Design review of the part built by this model. Coordinates are the model's own, in mm. A direction names the side the tool comes from. Round coordinates to 2 decimals unless told otherwise and drop trailing zeros. Loops run counter-clockwise (first coordinate to the right, second up) from the corner with the lowest first, then second, coordinate; pieces in that order, holes last. Notation, with made-up numbers: M 60.5,3.5 L 102.5,3.5 A21 cw 102.5,40.5 Z; hole C 84,-23.5 d9. An arc over 180 degrees is marked long. Use a Markdown table: item, result.
from build123d import *

# Parameters (mm, degrees)
SKETCH1_R           = 16
BOSS_EXTRUDE1_DEPTH = 12.5
SKETCH2_R           = 15
CUT_EXTRUDE1_DEPTH  = 10
SKETCH3_R           = 5
CUT_EXTRUDE2_DEPTH  = 10
SKETCH4_R           = 1
CUT_EXTRUDE3_DEPTH  = 10


with BuildPart() as part:
    # Sketch1 → Boss-Extrude1 (new body)
    with BuildSketch(Plane(origin=(0, 0, 0), x_dir=(1, 0, 0), z_dir=(0, 1, 0))):
        with Locations(Location((0, 0, 0), (0, 0, 270))):
            Circle(SKETCH1_R)
    extrude(amount=BOSS_EXTRUDE1_DEPTH)

    # Sketch2 → Cut-Extrude1 (cut)
    with BuildSketch(Plane(origin=(0, 12.5, 0), x_dir=(1, 0, 0), z_dir=(0, 1, 0))):
        with Locations(Location((0, 0, 0), (0, 0, 270))):
            Circle(SKETCH2_R)
    extrude(amount=-CUT_EXTRUDE1_DEPTH, mode=Mode.SUBTRACT)

    # Sketch3 → Cut-Extrude2 (cut)
    with BuildSketch(Plane(origin=(0, 0, 0), x_dir=(-1, 0, 0), z_dir=(0, -1, 0))):
        with Locations(Location((0, 0, 0), (0, 0, 90))):
            Circle(SKETCH3_R)
    extrude(amount=-CUT_EXTRUDE2_DEPTH, mode=Mode.SUBTRACT)

    # Sketch4 → Cut-Extrude3 (cut)
    with BuildSketch(Plane(origin=(0, 0, 0), x_dir=(-1, 0, 0), z_dir=(0, -1, 0))):
        with Locations(Location((0, 8, 0), (0, 0, 90))):
            Circle(SKETCH4_R)
        with Locations(Location((0, -8, 0), (0, 0, 90))):
            Circle(SKETCH4_R)
        with Locations(Location((-8, 0, 0), (0, 0, 90))):
            Circle(SKETCH4_R)
        with Locations(Location((8, 0, 0), (0, 0, 90))):
            Circle(SKETCH4_R)
    extrude(amount=-CUT_EXTRUDE3_DEPTH, mode=Mode.SUBTRACT)


solid = part.part
1. Insertion check: pin 1 (4 mm diameter, centred on x = 2.5, z = 7.5, fed in from +Y); pin 2 (6 mm diameter, centred on y = 4, z = 11, fed in from +X); pin 3 (1.2 mm diameter, centred on x = 0, z = 8, fed in from +Y); pin 4 (1.5 mm diameter, centred on x = -7.5, y = 9, fed in from +Z). Each pin has a flat end and moves straight along its axis. Give the tip position at first contact, or say it passes through.
Check values:
| item | result |
|---|---|
| pin 1 | stops at y = 2.5 |
| pin 2 | stops at x = 13.86 |
| pin 3 | passes through |
| pin 4 | stops at z = 14.51 |
2. Wall thickness on line 1 along X through (y, z) = (1.4, 0); line 2 along X through (y, z) = (5.5, 0); line 3 along Y through (x, z) = (3.5, 7): over which ranges is each line inside the solid? List them lowest first. Write a range as from..to.
Check values:
| item | result |
|---|---|
| line 1 | x = -16..-9, -7..-5, 5..7, 9..16 |
| line 2 | x = -16..-15, 15..16 |
| line 3 | y = 0..2.5 |
3. Take a section at B-B on z = -8. Give the boundary of the cut face in (x, y), and give its area (3 significant figures).
Check values:
| item | result |
|---|---|
| outline | M -13.86,0 L -1,0 L -1,2.5 L -12.69,2.5 L -12.69,12.5 L -13.86,12.5 Z; M 1,0 L 13.86,0 L 13.86,12.5 L 12.69,12.5 L 12.69,2.5 L 1,2.5 Z |
| area | 87.6 mm² |
4. Take a section at D-D on z = 6. Give the boundary of the cut face in (x, y).
Check values:
| item | result |
|---|---|
| outline | M -14.83,0 L 14.83,0 L 14.83,12.5 L 13.75,12.5 L 13.75,2.5 L -13.75,2.5 L -13.75,12.5 L -14.83,12.5 Z |
5. Machinability: for faces 4 (the face through (0.66, 7.57, -14.985)), 5 (the face through (9, 1, 0)), which of the approach directions +Z, -Z, +X, -X, +Y, -Y give a long, thin tool a straight path to every point of the face, cutting with its end or side? Answer none if there is none.
Check values:
| item | result |
|---|---|
| face 4 | +Y |
| face 5 | +Y, -Y |
6. Take a section at A-A on x = 0. Give the boundary of the cut face in (y, z), and give its area (3 significant figures).
Check values:
| item | result |
|---|---|
| outline | M 0,-16 L 12.5,-16 L 12.5,-15 L 2.5,-15 L 2.5,-9 L 0,-9 Z; M 0,-7 L 2.5,-7 L 2.5,-5 L 0,-5 Z; M 0,5 L 2.5,5 L 2.5,7 L 0,7 Z; M 0,9 L 2.5,9 L 2.5,15 L 12.5,15 L 12.5,16 L 0,16 Z |
| area | 65.0 mm² |
7. The part is to be moulded in two halves that separate along Z. For faces 1 (the face through (-15.62, 6.16, -3.47)), 2 (the face through (4, 0, -4)), 3 (the face through (-0.6, 1.2, 8.8)), say which applies: pulls with the +Z half, pulls with the -Z half, needs draft (parallel to the pull), parting line crosses it, or undercut.
Check values:
| item | result |
|---|---|
| face 1 | parting line crosses it |
| face 2 | needs draft |
| face 3 | undercut |
8. Take a section at C-C on x = -8. Give the boundary of the cut face in (y, z), and give its area (3 significant figures).
Check values:
| item | result |
|---|---|
| outline | M 0,-13.86 L 12.5,-13.86 L 12.5,-12.69 L 2.5,-12.69 L 2.5,-1 L 0,-1 Z; M 0,1 L 2.5,1 L 2.5,12.69 L 12.5,12.69 L 12.5,13.86 L 0,13.86 Z |
| area | 87.6 mm² |
